The listing builds one solid part. Answer for the finished solid, in the listing's coordinates (mm). Face numbers are marked on the shaded views. A direction names the side the tool comes from. Round coordinates to 2 decimals unless told otherwise and drop trailing zeros. Write each loop counter-clockwise with the first axis right and the second up, starting at its lowest first coordinate (ties: lowest second). Pieces come first, ordered by that corner, then holes.
from build123d import *

# Parameters (mm, degrees)
F1_DEPTH      = 10
F2_T1_DEPTH   = 34.4948974279
F3_R          = 1
F4_SCALE      = 0.5
F5_R          = 1
F6_DEPTH      = 25
F6_DEPTH_BACK = 25


# Not quite as in the source:
# - a fillet or chamfer that OpenCascade refuses, or shapes differently, is made with other operations: its cross-section is extruded or revolved along the edge and cut away or added


with BuildPart() as f1:
    # F0 (on Front) → F1 (new body)
    with BuildSketch(Plane.XZ):
        with BuildLine():
            Line((-11, 11.2686367076), (-11, 16.3676562212))
            Line((-11, 16.3676562212), (0, 16.3676562212))
            Line((0, 16.3676562212), (0, 11.2686367076))
            ThreePointArc((0, 11.2686367076), (1.4821200219, 13.6290434337), (2, 16.3676562212))
            ThreePointArc((2, 16.3676562212), (-8.2386127875, 23.3497762431), (-11, 11.2686367076))
        make_face()
        with BuildLine():
            Line((0, 16.3676562212), (-11, 16.3676562212))
            Line((-11, 16.3676562212), (-11, 11.2686367076))
            ThreePointArc((-11, 11.2686367076), (-5.5, 8.8676562212), (0, 11.2686367076))
            Line((0, 11.2686367076), (0, 16.3676562212))
        make_face()
        with BuildLine():
            ThreePointArc((0, 11.2686367076), (-5.5, 8.8676562212), (-11, 11.2686367076))
            Line((-11, 11.2686367076), (-11, 10.6633629519))
            Line((-11, 10.6633629519), (-11, 6.6633629519))
            Line((-11, 6.6633629519), (-11, -3.3366370481))
            Line((-11, -3.3366370481), (-11, -13.6323437788))
            Line((-11, -13.6323437788), (-6, -13.6323437788))
            Line((-6, -13.6323437788), (-6, -4.1323437788))
            Line((-6, -4.1323437788), (-5, -4.1323437788))
            Line((-5, -4.1323437788), (-5, -13.6323437788))
            Line((-5, -13.6323437788), (0, -13.6323437788))
            Line((0, -13.6323437788), (0, -3.3363437788))
            Line((0, -3.3363437788), (0, 6.6636562212))
            Line((0, 6.6636562212), (0, 10.6636562212))
            Line((0, 10.6636562212), (0, 11.2686367076))
        make_face()
        Polygon((-11, 6.6633629519), (-11, 10.6633629519), (-15, 10.6633629519), (-15, -3.3366370481), (-12, -3.3366370481), (-12, 6.6633629519), align=None)
        Polygon((4, 10.6636562212), (0, 10.6636562212), (0, 6.6636562212), (1, 6.6636562212), (1, -3.3363437788), (4, -3.3363437788), align=None)
    extrude(amount=F1_DEPTH)

    # F2: fillet of radius 5 on 2 edges, made by hand

    # F2_s2 → F2_t1 (cut)
    with BuildSketch(Plane.XZ.offset(-12.2474487139)):
        with BuildLine():
            ThreePointArc((4, 5.7646767356), (2.8729833462, 8.9269543958), (0, 10.6636562212))
            Line((0, 10.6636562212), (4, 10.6636562212))
            Line((4, 10.6636562212), (4, 5.7646767356))
        make_face()
        with BuildLine():
            ThreePointArc((-11, 10.6633629519), (-13.8729833462, 8.9266611265), (-15, 5.7643834664))
            Line((-15, 5.7643834664), (-15, 10.6633629519))
            Line((-15, 10.6633629519), (-11, 10.6633629519))
        make_face()
    extrude(amount=F2_T1_DEPTH, mode=Mode.SUBTRACT)

    # F3
    f3_edges = [f1.edges().sort_by_distance(p)[0] for p in [
        (-15, -5, -3.336637),
        (-12, -5, -3.336637),
        (1, -5, -3.336344),
        (4, -5, -3.336344),
        (-5, -5, -13.632344),
        (0, -5, -13.632344),
        (-11, -5, -13.632344),
        (-6, -5, -13.632344),
    ]]
    fillet(f3_edges, radius=F3_R)


with BuildPart() as f1_1:
    # F4: moved
    add(f1.part.scale(F4_SCALE))

    # F5 (on Right) → F6 (cut, two sides)
    with BuildSketch(Plane.YZ) as f6_sk:
        with Locations((-2.5, 8.6343183538)):
            Circle(F5_R)
    extrude(amount=-F6_DEPTH, mode=Mode.SUBTRACT)
    extrude(f6_sk.sketch, amount=F6_DEPTH_BACK, mode=Mode.SUBTRACT)


solid = f1_1.part
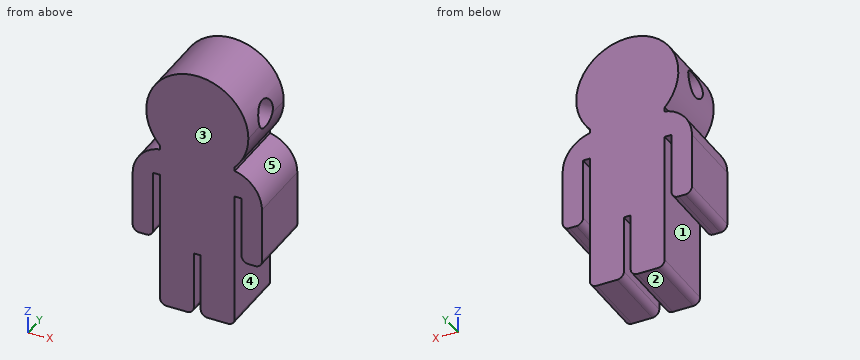
1. For a pull along X with two mould halves and no side action, classify the marked faces 3, 4 and 5 as released by +X, released by -X, zero draft, split by the parting line, or undercut.
Geometry says:
face 3: zero draft
face 4: undercut
face 5: released by +X
2. Straight lines are drawn through the part: line 1 along X through (y, z) = (-3.75, 1.5); line 2 along X through (y, z) = (-3.9, -3.25); line 3 along Z through (x, y) = (-2.75, -2.5). For each, find the intervals that lie inside material, in ascending order.
Geometry says:
line 1: x = -7.5 to -6, -5.5 to 0, 0.5 to 2
line 2: x = -5.5 to -3, -2.5 to 0
line 3: z = -2.07 to 7.63, 9.63 to 11.93
3. A tool of negligible diameter and unlimited length cuts with its end or side. For the marked faces 1 and 2, from which of +Z, -Z, +X, -X, +Y, -Y can it reach the whole face along a straight path? Write none if from no direction.
Geometry says:
face 1: -Z, +Y, -Y
face 2: -Z, +X, -X, +Y, -Y
4. Section D-D on y = -4.45 is taken. Determine the outline of the cut face in (x, z), plus the area to 3 significant figures.
Geometry says:
outline: (-7.5, -1.17) arc R0.5 ccw to (-7, -1.67) - (-6.5, -1.67) arc R0.5 ccw to (-6, -1.17) - (-6, 3.33) - (-5.5, 3.33) - (-5.5, -6.32) arc R0.5 ccw to (-5, -6.82) - (-3.5, -6.82) arc R0.5 ccw to (-3, -6.32) - (-3, -2.07) - (-2.5, -2.07) - (-2.5, -6.32) arc R0.5 ccw to (-2, -6.82) - (-0.5, -6.82) arc R0.5 ccw to (0, -6.32) - (0, 3.33) - (0.5, 3.33) - (0.5, -1.17) arc R0.5 ccw to (1, -1.67) - (1.5, -1.67) arc R0.5 ccw to (2, -1.17) - (2, 2.88) arc R2.5 ccw to (0, 5.33) - (0, 5.63) arc R3.75 ccw (long way) to (-5.5, 5.63) - (-5.5, 5.33) arc R2.5 ccw to (-7.5, 2.88) - close
area: 126 mm2
5. Section A-A on z = 1.5 is taken. Determine the outline of the cut face in (x, y).
Geometry says:
outline: (-7.5, -5) - (-6, -5) - (-6, 0) - (-7.5, 0) - close; (-5.5, -5) - (0, -5) - (0, 0) - (-5.5, 0) - close; (0.5, -5) - (2, -5) - (2, 0) - (0.5, 0) - close
6. Given pin 1 (1.2 mm diameter, centred on y = -2.5, z = 8.63, fed in from +X); pin 2 (3 mm diameter, centred on y = -2.5, z = 8.63, fed in from -X); pin 3 (2 mm diameter, centred on y = -2.5, z = -4, fed in from +X); pin 4 (1 mm diameter, centred on x = -5, y = -2.5, fed in from +Z), each flat-ended and moving along its own axis, determine where each tip first touches the part or whether it passes through.
Geometry says:
pin 1: passes through
pin 2: stops at x = -6.5
pin 3: stops at x = 0
pin 4: stops at z = 11.5
7. Section C-C on z = -4.5 is taken. Determine the outline of the cut face in (x, y).
Geometry says:
outline: (-5.5, -5) - (-3, -5) - (-3, 0) - (-5.5, 0) - close; (-2.5, -5) - (0, -5) - (0, 0) - (-2.5, 0) - close
